```python
from build123d import *

# Parameters (mm, degrees)
SKETCH_1_W          = 120
SKETCH_1_H          = 280
SKETCH_1_R          = 4.25
EXTRUDE_1_DEPTH     = 10
FILLET_1_R          = 5
SKETCH_2_W          = 120
SKETCH_2_H          = 100
EXTRUDE_2_DEPTH     = 2
SKETCH_3_R          = 4.25
CUT_EXTRUDE_1_DEPTH = 35
SKETCH_5_R          = 7
CUT_EXTRUDE_3_DEPTH = 8.5


with BuildPart() as part:
    # 草图1 → 凸台-拉伸1 (new body)
    with BuildSketch(Plane.XY):
        Rectangle(SKETCH_1_W, SKETCH_1_H)
        with Locations((36, 25)):
            Circle(SKETCH_1_R, mode=Mode.SUBTRACT)
        with Locations(Location((36, -25, 0), (0, 0, 180))):
            Circle(SKETCH_1_R, mode=Mode.SUBTRACT)
        with Locations((-36, -25)):
            Circle(SKETCH_1_R, mode=Mode.SUBTRACT)
        with Locations(Location((-36, 25, 0), (0, 0, 180))):
            Circle(SKETCH_1_R, mode=Mode.SUBTRACT)
    extrude(amount=EXTRUDE_1_DEPTH)

    # 圆角1
    fillet_1_edges = [part.edges().sort_by_distance(p)[0] for p in [
        (-60, 140, 5),
        (60, 140, 5),
        (60, -140, 5),
        (-60, -140, 5),
    ]]
    fillet(fillet_1_edges, radius=FILLET_1_R)

    # 草图2 → 凸台-拉伸2 (add)
    with BuildSketch(Plane.XY.offset(10)):
        Rectangle(SKETCH_2_W, SKETCH_2_H)
    extrude(amount=EXTRUDE_2_DEPTH)

    # 草图3 → 切除-拉伸1 (cut)
    with BuildSketch(Plane(origin=(0, 0, 0), x_dir=(-1, 0, 0), z_dir=(0, 0, -1))):
        with Locations((-36, -25)):
            Circle(SKETCH_3_R)
        with Locations((-36, 25)):
            Circle(SKETCH_3_R)
        with Locations((36, 25)):
            Circle(SKETCH_3_R)
        with Locations((36, -25)):
            Circle(SKETCH_3_R)
    extrude(amount=-CUT_EXTRUDE_1_DEPTH, mode=Mode.SUBTRACT)

    # 草图5 → 切除-拉伸3 (cut)
    with BuildSketch(Plane(origin=(0, 0, 0), x_dir=(-1, 0, 0), z_dir=(0, 0, -1))):
        with Locations((36, 25)):
            Circle(SKETCH_5_R)
        with Locations((36, -25)):
            Circle(SKETCH_5_R)
        with Locations((-36, -25)):
            Circle(SKETCH_5_R)
        with Locations((-36, 25)):
            Circle(SKETCH_5_R)
    extrude(amount=-CUT_EXTRUDE_3_DEPTH, mode=Mode.SUBTRACT)


solid = part.part
```
Source: CAD feature listing. Evaluate the final solid. Frame: model axes, mm. A direction names the side the tool comes from. Round coordinates to 2 decimals unless told otherwise and drop trailing zeros. Loops run counter-clockwise (first coordinate to the right, second up) from the corner with the lowest first, then second, coordinate; pieces in that order, holes last.
(1) Material intervals for probe 1 along X at (y, z) = (-25, 10.75); probe 2 along Y at (x, z) = (-36, 6.75); probe 3 along Y at (x, z) = (-36, 10.8), sorted ascending.
From the geometry:
probe 1: x = -60 to -40.25, -31.75 to 31.75, 40.25 to 60
probe 2: y = -140 to -32, -18 to 18, 32 to 140
probe 3: y = -50 to -29.25, -20.75 to 20.75, 29.25 to 50
(2) Section query B-B (z = 5). Output: boundary loops of the cut face in (x, y).
From the geometry:
outline: (-60, -135) arc R5 ccw to (-55, -140) - (55, -140) arc R5 ccw to (60, -135) - (60, 135) arc R5 ccw to (55, 140) - (-55, 140) arc R5 ccw to (-60, 135) - close; hole circle Ø14 at (-36, -25); hole circle Ø14 at (-36, 25); hole circle Ø14 at (36, -25); hole circle Ø14 at (36, 25)
(3) Contact query for flat-ended pins moving along their axis: pin 1 Ø4 at (x, y) = (-36, -27.5) entering from -Z; pin 2 Ø1.6 at (x, z) = (-28, 11.5) entering from +Y. Output: stop coordinate, or through.
From the geometry:
pin 1: stops at z = 8.5
pin 2: stops at y = 50
(4) Section query C-C (x = 26). Output: boundary loops of the cut face in (y, z), and give its area (3 significant figures).
From the geometry:
outline: (-140, 0) - (140, 0) - (140, 10) - (50, 10) - (50, 12) - (-50, 12) - (-50, 10) - (-140, 10) - close
area: 3,000 mm2
(5) Section query D-D (y = -92). Output: boundary loops of the cut face in (x, z), and give its area (3 significant figures).
From the geometry:
outline: (-60, 0) - (60, 0) - (60, 10) - (-60, 10) - close
area: 1,200 mm2
(6) Access query for faces 5 (the flat face through (-1, -94, 10)), 6 (the cylindrical face through (32.77, -31.21, 4.19)), 7 (the flat face through (-1, -140, 5)). Directions: +Z, -Z, +X, -X, +Y, -Y. A direction counts if a zero-diameter tool reaches every point of the face in a straight line with its end or side. Return the directions, or none.
From the geometry:
face 5: +Z, +X, -X, -Y
face 6: -Z
face 7: +Z, -Z, +X, -X, -Y
(7) Section query A-A (x = -36). Output: boundary loops of the cut face in (y, z).
From the geometry:
outline: (-140, 0) - (-32, 0) - (-32, 8.5) - (-29.25, 8.5) - (-29.25, 12) - (-50, 12) - (-50, 10) - (-140, 10) - close; (-20.75, 8.5) - (-18, 8.5) - (-18, 0) - (18, 0) - (18, 8.5) - (20.75, 8.5) - (20.75, 12) - (-20.75, 12) - close; (29.25, 8.5) - (32, 8.5) - (32, 0) - (140, 0) - (140, 10) - (50, 10) - (50, 12) - (29.25, 12) - close
(8) Pull-direction query (Y, two-part tool) for faces 1 (the flat face through (36, -30, 8.5)), 2 (the flat face through (36, 20, 8.5)), 3 (the flat face through (-1, 96, 10)), 4 (the cylindrical face through (58, -139, 5)); classes: +Y half, -Y half, draft (parallel to the pull), parting line (faces both ways), or undercut.
From the geometry:
face 1: undercut
face 2: undercut
face 3: draft
face 4: -Y half
